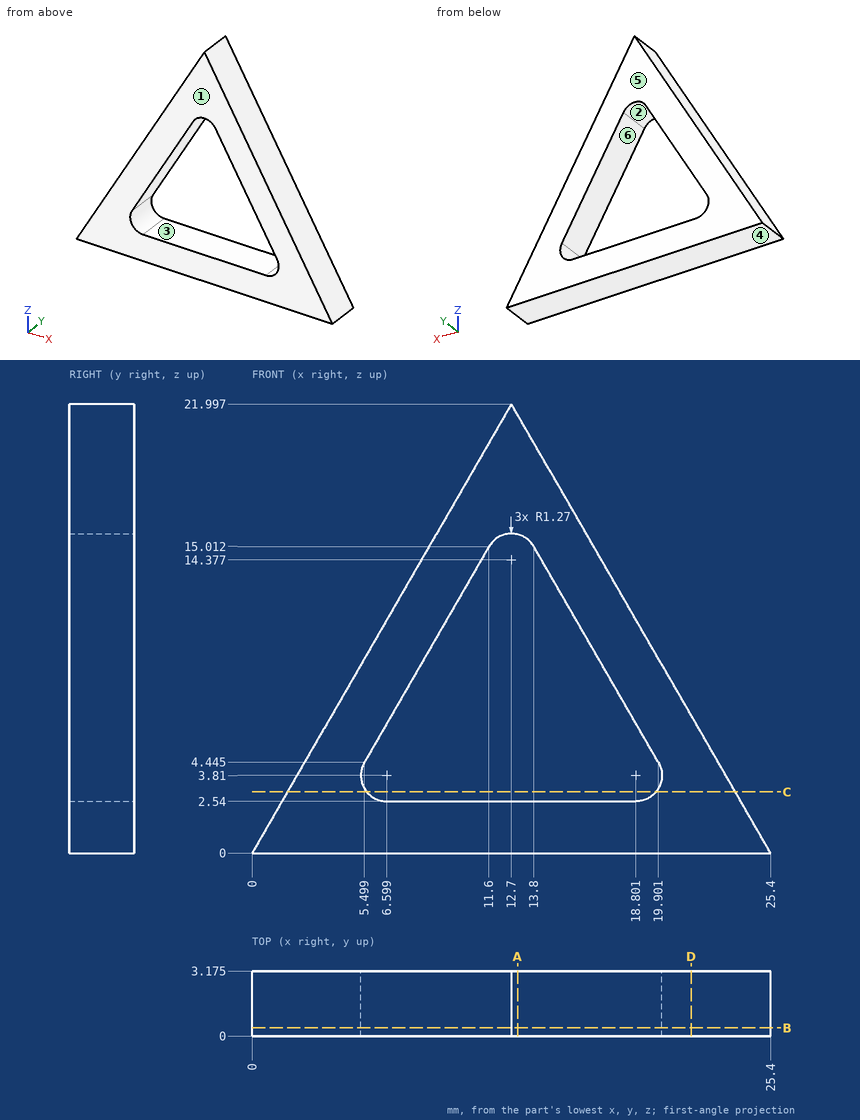
Input: dimensioned drawing with shaded views. Units: mm. Origin: part minimum x, y, z. A direction names the side the tool comes from. Coordinates: 2 decimals unless noted, no trailing zeros. Order: outer loops, then holes, each group sorted by start corner. A loop starts at its lowest first (then second) coordinate and runs counter-clockwise, first axis right, second up.
(1) Access query for the marked faces 5 and 6. Directions: +Z, -Z, +X, -X, +Y, -Y. A direction counts if a zero-diameter tool reaches every point of the face in a straight line with its end or side. Return the directions, or none.
(2) Section query D-D (x = 21.5). Return the cut outline in (y, z) (1 decimal).
(3) Section query A-A (x = 13). Return the cut outline in (y, z) (1 decimal).
(4) Material intervals for probe 1 along X at (y, z) = (2.7, 8.5); probe 2 along Z at (x, y) = (7.25, 1.85); probe 3 along Z at (x, y) = (14.25, 1.5), sorted ascending.
(5) Draft query along Z for the marked faces 1, 2, 3 and 4. Return one class per face: pulls with the +Z half, pulls with the -Z half, needs draft (parallel to the pull), parting line crosses it, or undercut.
(6) Section query B-B (y = 0.4). Return the cut outline in (x, z) (1 decimal).
(7) Section query C-C (z = 3). Return the cut outline in (x, y) (1 decimal).
Solution:
1. face 5: +Z, -Z, +X, -X, +Y
1. face 6: +Y, -Y
2. outline: (0, 0) - (3.2, 0) - (3.2, 6.8) - (0, 6.8) - close
3. outline: (0, 0) - (3.2, 0) - (3.2, 2.5) - (0, 2.5) - close; (0, 15.6) - (3.2, 15.6) - (3.2, 21.5) - (0, 21.5) - close
4. probe 1: x = 4.91 to 7.84, 17.56 to 20.49
4. probe 2: z = 0 to 2.54, 7.48 to 12.56
4. probe 3: z = 0 to 2.54, 14.23 to 19.31
5. face 1: needs draft
5. face 2: undercut
5. face 3: undercut
5. face 4: pulls with the -Z half
6. outline: (0, 0) - (25.4, 0) - (12.7, 22) - close; hole (5.5, 4.4) arc R1.3 ccw to (6.6, 2.5) - (18.8, 2.5) arc R1.3 ccw to (19.9, 4.4) - (13.8, 15) arc R1.3 ccw to (11.6, 15) - close
7. outline: (1.7, 0) - (5.6, 0) - (5.6, 3.2) - (1.7, 3.2) - close; (19.8, 0) - (23.7, 0) - (23.7, 3.2) - (19.8, 3.2) - close
